from build123d import *

# Parameters (mm, degrees)
F1_W     = 330.2
F1_H     = 101.6
F1_R     = 8.73125
F1_R_2   = 3.397434
F2_DEPTH = 5


with BuildPart() as f2:
    # F1 (on Front) → F2 (new body)
    with BuildSketch(Plane.XZ):
        Rectangle(F1_W, F1_H)
        with Locations((-114.3, -26.9875)):
            Circle(F1_R, mode=Mode.SUBTRACT)
        with Locations((-98.536217, -27.303673)):
            Circle(F1_R_2, mode=Mode.SUBTRACT)
        with Locations((-137.671861, -13.49375)):
            Circle(F1_R, mode=Mode.SUBTRACT)
        with Locations((-122.181891, -13.651836)):
            Circle(F1_R_2, mode=Mode.SUBTRACT)
        with Locations((-106.418109, -13.651836)):
            Circle(F1_R_2, mode=Mode.SUBTRACT)
        with Locations((-90.928139, -13.49375)):
            Circle(F1_R, mode=Mode.SUBTRACT)
        with Locations((-130.063783, 0)):
            Circle(F1_R_2, mode=Mode.SUBTRACT)
        with Locations((-114.3, 0)):
            Circle(F1_R, mode=Mode.SUBTRACT)
        with Locations((-98.536217, 0)):
            Circle(F1_R_2, mode=Mode.SUBTRACT)
        with Locations((-82.772434, 0)):
            Circle(F1_R_2, mode=Mode.SUBTRACT)
        with Locations((114.3, -26.9875)):
            Circle(F1_R, mode=Mode.SUBTRACT)
        with Locations((130.063783, -27.303673)):
            Circle(F1_R_2, mode=Mode.SUBTRACT)
        with Locations((90.928139, -13.49375)):
            Circle(F1_R, mode=Mode.SUBTRACT)
        with Locations((106.418109, -13.651836)):
            Circle(F1_R_2, mode=Mode.SUBTRACT)
        with Locations((122.181891, -13.651836)):
            Circle(F1_R_2, mode=Mode.SUBTRACT)
        with Locations((137.671861, -13.49375)):
            Circle(F1_R, mode=Mode.SUBTRACT)
        with Locations((98.536217, 0)):
            Circle(F1_R_2, mode=Mode.SUBTRACT)
        with Locations((114.3, 0)):
            Circle(F1_R, mode=Mode.SUBTRACT)
        with Locations((130.063783, 0)):
            Circle(F1_R_2, mode=Mode.SUBTRACT)
        with Locations((145.827566, 0)):
            Circle(F1_R_2, mode=Mode.SUBTRACT)
        with Locations((-137.671861, 13.49375)):
            Circle(F1_R, mode=Mode.SUBTRACT)
        with Locations((-122.181891, 13.651836)):
            Circle(F1_R_2, mode=Mode.SUBTRACT)
        with Locations((-106.418109, 13.651836)):
            Circle(F1_R_2, mode=Mode.SUBTRACT)
        with Locations((-90.928139, 13.49375)):
            Circle(F1_R, mode=Mode.SUBTRACT)
        with Locations((-114.3, 26.9875)):
            Circle(F1_R, mode=Mode.SUBTRACT)
        with Locations((-98.536217, 27.303673)):
            Circle(F1_R_2, mode=Mode.SUBTRACT)
        with Locations((90.928139, 13.49375)):
            Circle(F1_R, mode=Mode.SUBTRACT)
        with Locations((106.418109, 13.651836)):
            Circle(F1_R_2, mode=Mode.SUBTRACT)
        with Locations((122.181891, 13.651836)):
            Circle(F1_R_2, mode=Mode.SUBTRACT)
        with Locations((137.671861, 13.49375)):
            Circle(F1_R, mode=Mode.SUBTRACT)
        with Locations((114.3, 26.9875)):
            Circle(F1_R, mode=Mode.SUBTRACT)
        with Locations((130.063783, 27.303673)):
            Circle(F1_R_2, mode=Mode.SUBTRACT)
    extrude(amount=F2_DEPTH)


solid = f2.part
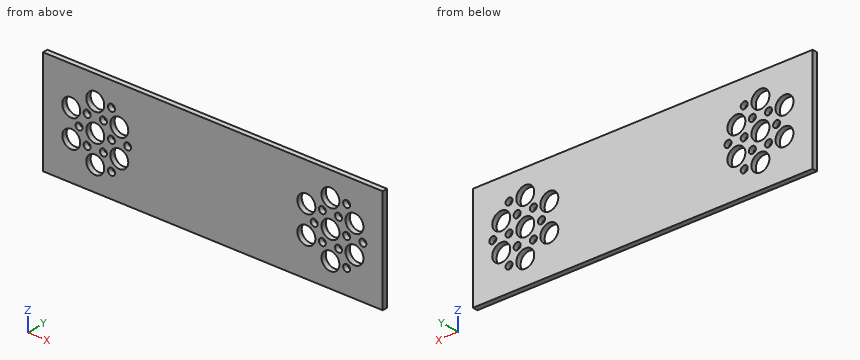
The listing builds one solid part. Answer for the finished solid, in the listing's coordinates (mm). Give positions to 0.01 mm unless a question says otherwise; leave off trailing zeros. Order: outer loops, then holes, each group sorted by start corner. A loop starts at its lowest first (then second) coordinate and runs counter-clockwise, first axis right, second up. Notation, with made-up numbers: (-22.5, 19.25) - (3.5, 19.25) arc R15 ccw to (3.5, 42.25) - close; hole circle Ø2 at (-18.75, 68.25). An arc over 180 degrees is marked (long way). Answer as CSV lines item,"result".
Q1. A cutting plane is placed at B-B, the plane z = 0. Count the separate pieces of the cut face and the enclosed holes in it, and give its area (3 significant figures).
Answer key:
separate pieces,"9"
enclosed holes,"0"
area,"1,270 mm^2"
Q2. A cutting plane is placed at A-A, the plane x = -114.3. Determine the outline of the cut face in (y, z).
Answer key:
outline,"(-5, -50.8) - (0, -50.8) - (0, -35.72) - (-5, -35.72) - close; (-5, -18.26) - (0, -18.26) - (0, -8.73) - (-5, -8.73) - close; (-5, 8.73) - (0, 8.73) - (0, 18.26) - (-5, 18.26) - close; (-5, 35.72) - (0, 35.72) - (0, 50.8) - (-5, 50.8) - close"
Q3. Straight lines are drawn through the part: L1, parallel to Z at x = -114.3, y = -3; L2, parallel to Z at x = 107, y = -4.05; L3, parallel to Z at x = -101, y = -2.85. For each, find the intervals that lie inside material, in ascending order.
Answer key:
L1,"z = -50.8 to -35.72, -18.26 to -8.73, 8.73 to 18.26, 35.72 to 50.8"
L2,"z = -50.8 to -31.78, -22.2 to -17, -10.3 to -4.79, 4.79 to 10.3, 17 to 22.2, 31.78 to 50.8"
L3,"z = -50.8 to -29.64, -24.96 to -2.34, 2.34 to 24.96, 29.64 to 50.8"
Q4. This flat-tipped pin is pushed along its axis until it touches: pin 1 Ø5.5 at (x, z) = (-122.18, 13.65) entering from -Y. Where does it stop, or does it pass through?
Answer key:
pin 1,"passes through"
